Input: dimensioned drawing with shaded views. Units: mm. Origin: part minimum x, y, z. Coordinates: 2 decimals unless noted, no trailing zeros. Loops run counter-clockwise (first coordinate to the right, second up) from the corner with the lowest first, then second, coordinate; pieces in that order, holes last.
Item 1: Section A-A on z = 10. Return loops of the section in (x, y), and give its area (3 significant figures).
Item 2: Contact query for a flat-ended pin moving along its axis: P1, Ø1.5, axis at x = 22.5, z = 10.5, coming from the +Y side. Output: stop coordinate, or through.
Item 3: Section B-B on x = 22.5. Return loops of the section in (y, z), and give its area (3 significant figures).
Item 4: Ray query, line 1 along X through (y, z) = (6, 10); line 2 along Y through (x, z) = (15, 19.25); line 3 along Z through (x, y) = (7.5, 5.7). Return the intervals inside material, ascending.
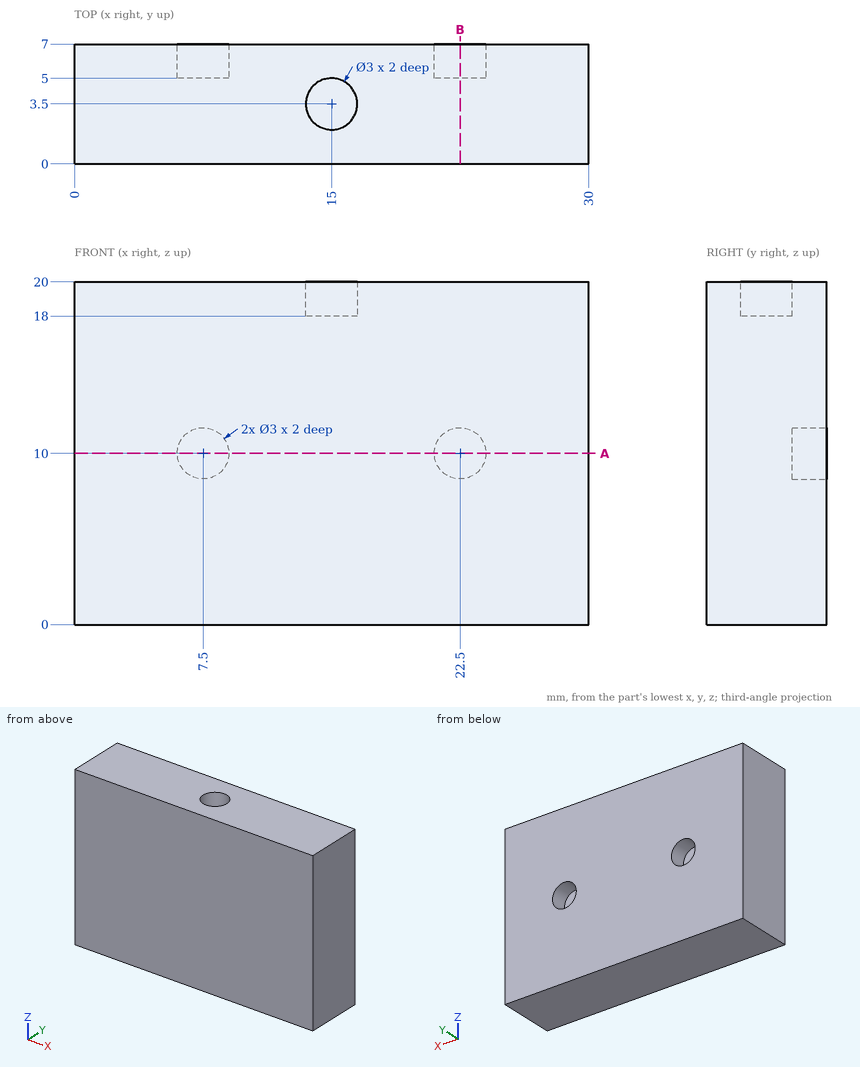
Results found:
1. outline: (0, 0) - (30, 0) - (30, 7) - (24, 7) - (24, 5) - (21, 5) - (21, 7) - (9, 7) - (9, 5) - (6, 5) - (6, 7) - (0, 7) - close
1. area: 198 mm2
2. P1: stops at y = 5
3. outline: (0, 0) - (7, 0) - (7, 8.5) - (5, 8.5) - (5, 11.5) - (7, 11.5) - (7, 20) - (0, 20) - close
3. area: 134 mm2
4. line 1: x = 0 to 6, 9 to 21, 24 to 30
4. line 2: y = 0 to 2, 5 to 7
4. line 3: z = 0 to 8.5, 11.5 to 20
